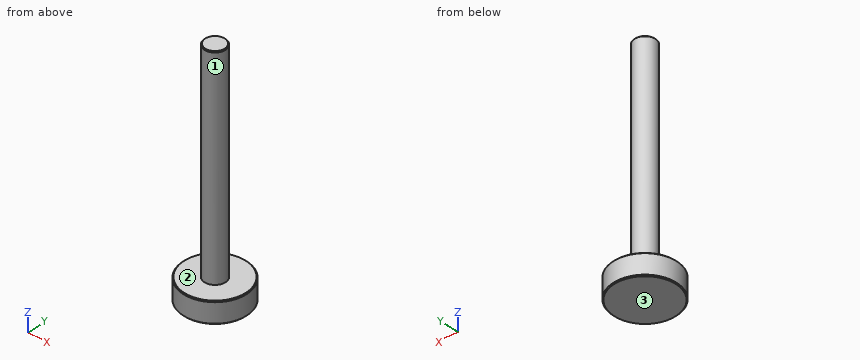
Autodesk Inventor part; units mm, degrees
ref_plane "YZ Plane" through (0, 0, 0) normal (1, 0, 0) x (0, 1, 0)
ref_plane "XZ Plane" through (0, 0, 0) normal (0, 1, 0) x (-1, 0, 0)
ref_plane "XY Plane" through (0, 0, 0) normal (0, 0, 1) x (1, 0, 0)
sketch "Sketch1" plane through (0, 0, 0) normal (0, 0, 1) x (1, 0, 0)
  circle A0 centre (0, 0) radius 9.525
extrude "Extrusion1" add sketch "Sketch1" along normal blind 6.35
sketch "Sketch2" plane through (0, 0, 6.35) normal (0, 0, 1) x (1, 0, 0)
  circle A0 centre (0, 0) radius 9.525
  circle A1 centre (0, 0) radius 3.175
extrude "Extrusion2" add sketch "Sketch2" along normal blind 63.5 contours A1
chamfer "Chamfer1" distance 0.254 angle 45 3 edges at (-3.175, 0, 69.85) (-9.525, 0, 6.35) (-9.525, 0, 0)
properties part number "piston_rod"
Verification items for the finished model (mm, model axes). Face numbers are marked on the shaded views. Round coordinates to 2 decimals unless told otherwise and drop trailing zeros. Loops run counter-clockwise (first coordinate to the right, second up) from the corner with the lowest first, then second, coordinate; pieces in that order, holes last. Notation, with made-up numbers: (-29.5, 2) - (23.5, 2) arc R21 ccw to (23.5, 19) - close; hole circle Ø7 at (46.25, -32.75). An arc over 180 degrees is marked (long way). Use a Markdown table: item, result. Add a question column.
1. Section check C-C, the plane z = 46. Record the boundary of the cut face in (x, y) (3 decimals).
2. Section check A-A, the plane y = 0. Record the boundary of the cut face in (x, z) (3 decimals).
3. Gauge pin test, flat ends, axial feed: pin 1 (4 mm diameter, centred on x = -3.5, z = 33, fed in from -Y); pin 2 (1 mm diameter, centred on y = -3, z = 35, fed in from -X); pin 3 (6 mm diameter, centred on x = -1, z = 62.5, fed in from -Y) (3 decimals). Record the tip position at first contact, or that the pin passes through.
4. Thickness scan on probe 1 along Z at (x, y) = (2.75, -2); probe 2 along X at (y, z) = (-1.25, 51.5); probe 3 along X at (y, z) = (-1, 43). Record the ranges inside material, lowest first. Write a range as [from, to].
5. Release check for a two-part mould opening along Z. For the marked faces 1, 2 and 3 record: released by +Z, released by -Z, zero draft, split by the parting line, or undercut.
Checks:
| question | item | result |
|---|---|---|
| 1 | outline | circle Ø6.35 at (0, 0) |
| 2 | outline | (-9.525, 0.254) - (-9.271, 0) - (9.271, 0) - (9.525, 0.254) - (9.525, 6.096) - (9.271, 6.35) - (3.175, 6.35) - (3.175, 69.596) - (2.921, 69.85) - (-2.921, 69.85) - (-3.175, 69.596) - (-3.175, 6.35) - (-9.271, 6.35) - (-9.525, 6.096) - close |
| 3 | pin 1 | stops at y = -2.8 |
| 3 | pin 2 | stops at x = -1.96 |
| 3 | pin 3 | stops at y = -3.175 |
| 4 | probe 1 | z = [0, 6.35] |
| 4 | probe 2 | x = [-2.92, 2.92] |
| 4 | probe 3 | x = [-3.01, 3.01] |
| 5 | face 1 | zero draft |
| 5 | face 2 | released by +Z |
| 5 | face 3 | released by -Z |
